Model file for the job. Use its own axes, mm. A direction names the side the tool comes from. Coordinates: 2 decimals unless noted, no trailing zeros. Write each loop counter-clockwise with the first axis right and the second up, starting at its lowest first coordinate (ties: lowest second). Pieces come first, ordered by that corner, then holes. Notation, with made-up numbers: M -38.75,-38.75 L -0.75,-38.75 A18 cw -0.75,-7.75 Z; hole C 75.25,30.5 d3. An arc over 180 degrees is marked long. Put each result on its own line as item: value. Start each with the question number.
Q1. Drop flat-ended pins along their axis: pin 1 (8 mm diameter, centred on x = 11.5, y = -18, fed in from +Z); pin 2 (4.5 mm diameter, centred on y = -70, z = 10, fed in from +X). Give the stop position or say it passes through.
Q2. Cut at B-B (x = 8.5). Write the cut outline in (y, z), then the cut area to 3 significant figures.
Q3. Cut at C-C (y = -70). Write the cut outline in (x, z).
Q4. Which spindle directions (+Z, -Z, +X, -X, +Y, -Y) get a long thin tool onto all of the face, cutting with end or side? Do faces 4 (the flat face through (8, -39, 2)), 5 (the cylindrical face through (1, -68, 8.5)). Say none if no direction does.
Q5. Cut at A-A (z = 10). Write the cut outline in (x, y), then the cut area to 3 significant figures.
Q6. Drill centre lines: line 1 along Z through (x, y) = (1.45, -70); line 2 along Y through (x, z) = (10, 1.05); line 3 along X through (y, z) = (-52, 2.75). Where is each one in solid material? Low to high.
Q7. Pull direction X, two halves, no side cores. Call faces 1 (the flat face through (7, -39, 0)), 2 (the flat face through (2, -41, 9)), 3 (the cylindrical face through (9.46, -12.44, 1.01)): pulls with the +X half, pulls with the -X half, needs draft (parallel to the pull), parting line crosses it, or undercut.
Q8. Cut at D-D (y = -47). Write the cut outline in (x, z).
```python
from build123d import *

# Parameters (mm, degrees)
ESQUISSE1_W             = 15
ESQUISSE1_H             = 80
BOSS_EXTRU_1_DEPTH      = 2
ESQUISSE2_W             = 2
ESQUISSE2_H             = 80
BOSS_EXTRU_2_DEPTH      = 15
ESQUISSE3_R             = 2.5
ENL_V_MAT_EXTRU_1_DEPTH = 20
ESQUISSE4_R             = 2.5
ENL_V_MAT_EXTRU_2_DEPTH = 20


with BuildPart() as part:
    # Esquisse1 → Boss.-Extru.1 (new body)
    with BuildSketch(Plane.XY):
        with Locations((7.5, -40)):
            Rectangle(ESQUISSE1_W, ESQUISSE1_H)
    extrude(amount=BOSS_EXTRU_1_DEPTH)

    # Esquisse2 → Boss.-Extru.2 (add)
    with BuildSketch(Plane.XY.offset(2)):
        with Locations((1, -40)):
            Rectangle(ESQUISSE2_W, ESQUISSE2_H)
    extrude(amount=BOSS_EXTRU_2_DEPTH)

    # Esquisse3 → Enlèv. mat.-Extru.1 (cut)
    with BuildSketch(Plane.XY.offset(2)):
        with Locations((10, -10)):
            Circle(ESQUISSE3_R)
    extrude(amount=-ENL_V_MAT_EXTRU_1_DEPTH, mode=Mode.SUBTRACT)

    # Esquisse4 → Enlèv. mat.-Extru.2 (cut)
    with BuildSketch(Plane.ZY):
        with Locations(Location((10, -70, 0), (0, 0, 270))):
            Circle(ESQUISSE4_R)
    extrude(amount=-ENL_V_MAT_EXTRU_2_DEPTH, mode=Mode.SUBTRACT)


solid = part.part
```
Computed values:
1. pin 1: z = 2
1. pin 2: through
2. outline: M -80,0 L -12,0 L -12,2 L -80,2 Z; M -8,0 L 0,0 L 0,2 L -8,2 Z
2. area: 152 mm2
3. outline: M 0,0 L 15,0 L 15,2 L 2,2 L 2,7.5 L 0,7.5 Z; M 0,12.5 L 2,12.5 L 2,17 L 0,17 Z
4. face 4: +Z, +X, +Y, -Y
4. face 5: +X, -X
5. outline: M 0,-80 L 2,-80 L 2,-72.5 L 0,-72.5 Z; M 0,-67.5 L 2,-67.5 L 2,0 L 0,0 Z
5. area: 150 mm2
6. line 1: 0 to 7.5, 12.5 to 17
6. line 2: -80 to -12.5, -7.5 to 0
6. line 3: 0 to 2
7. face 1: needs draft
7. face 2: pulls with the +X half
7. face 3: undercut
8. outline: M 0,0 L 15,0 L 15,2 L 2,2 L 2,17 L 0,17 Z
